Verification items for the finished model (mm, model axes). Face numbers are marked on the shaded views. A direction names the side the tool comes from. Round coordinates to 2 decimals unless told otherwise and drop trailing zeros. Write each loop counter-clockwise with the first axis right and the second up, starting at its lowest first coordinate (ties: lowest second). Pieces come first, ordered by that corner, then holes. Notation, with made-up numbers: (81.5, -37.5) -> (133.5, -37.5) arc R20 cw to (133.5, -0.5) -> close; hole circle Ø3 at (66, 57.5). An arc over 180 degrees is marked (long way). Answer as a JSON object with one key per item and string values. Group by question number.
(1) Sectioned sample at B-B on x = 29. Record the cut outline in (y, z).
(2) Scan lines: L1, parallel to X at y = -41, z = 7; L2, parallel to Y at x = -60, z = 83.5; L3, parallel to Y at x = 21, z = 69. Record each from-to range of solid material in increasing order. Write a range as from..to.
(3) Gauge pin test, flat ends, axial feed: pin 1 Ø3 at (y, z) = (-21, 25.5) entering from +X; pin 2 Ø2 at (y, z) = (14, 122.5) entering from -X; pin 3 Ø4 at (x, y) = (8, 21.5) entering from -Z; pin 4 Ø1 at (x, z) = (21.5, 25.5) entering from -Y. Record the tip position at first contact, or that the pin passes through.
(4) Sectioned sample at A-A on z = 19. Record the cut outline in (x, y).
(5) Set-up check for the marked faces 1, 2 and 3: record each of +Z, -Z, +X, -X, +Y, -Y from which the full face is reachable in a straight line by a thin tool's end or side.
(6) Sectioned sample at C-C on y = 39. Record the cut outline in (x, z).
```python
from build123d import *

# Parameters (mm, degrees)
F1_DEPTH = 146.05
F2_R     = 6.35


with BuildPart() as f1:
    # F0 (on Top) → F1 (new body)
    with BuildSketch(Plane.XY):
        Polygon((0, -52.3875), (0, -17.4625), (69.85, -17.4625), (69.85, 52.3875), (0, 52.3875), (0, 17.4625), (-69.85, 17.4625), (-69.85, -52.3875), align=None)
    extrude(amount=F1_DEPTH)

    # F2
    f2_edges = [f1.edges().sort_by_distance(p)[0] for p in [
        (-34.925, -52.3875, 146.05),
        (0, -34.925, 146.05),
        (34.925, -17.4625, 146.05),
        (69.85, 17.4625, 146.05),
        (34.925, 52.3875, 146.05),
        (0, 34.925, 146.05),
        (-34.925, 17.4625, 146.05),
        (-69.85, -17.4625, 146.05),
        (-69.85, -52.3875, 73.025),
        (0, -52.3875, 73.025),
        (-34.925, -52.3875, 0),
        (0, -17.4625, 73.025),
        (69.85, -17.4625, 73.025),
        (34.925, -17.4625, 0),
        (69.85, 52.3875, 73.025),
        (69.85, 17.4625, 0),
        (0, 52.3875, 73.025),
        (34.925, 52.3875, 0),
        (0, 17.4625, 73.025),
        (0, 34.925, 0),
        (-69.85, 17.4625, 73.025),
        (-34.925, 17.4625, 0),
        (-69.85, -17.4625, 0),
        (0, -34.925, 0),
    ]]
    fillet(f2_edges, radius=F2_R)


solid = f1.part
```
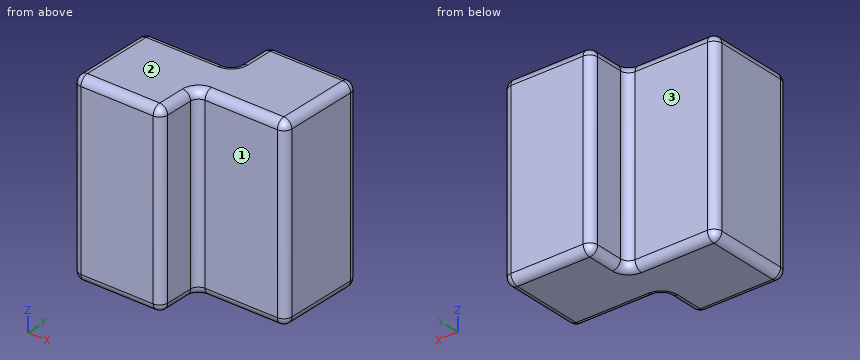
Computed values:
{
 "1": {"outline": "(-17.46, 6.35) arc R6.35 ccw to (-11.11, 0) -> (46.04, 0) arc R6.35 ccw to (52.39, 6.35) -> (52.39, 139.7) arc R6.35 ccw to (46.04, 146.05) -> (-11.11, 146.05) arc R6.35 ccw to (-17.46, 139.7) -> close"},
 "2": {"L1": "-69.85..0", "L2": "-52.39..17.46", "L3": "-17.46..52.39"},
 "3": {"pin 1": "x = 1.69", "pin 2": "x = -69.56", "pin 3": "z = 0", "pin 4": "y = -17.46"},
 "4": {"outline": "(-69.85, -46.04) arc R6.35 ccw to (-63.5, -52.39) -> (-6.35, -52.39) arc R6.35 ccw to (0, -46.04) -> (0, -23.81) arc R6.35 cw to (6.35, -17.46) -> (63.5, -17.46) arc R6.35 ccw to (69.85, -11.11) -> (69.85, 46.04) arc R6.35 ccw to (63.5, 52.39) -> (6.35, 52.39) arc R6.35 ccw to (0, 46.04) -> (0, 23.81) arc R6.35 cw to (-6.35, 17.46) -> (-63.5, 17.46) arc R6.35 ccw to (-69.85, 11.11) -> close"},
 "5": {"face 1": "+Z, -Z, +X, -Y", "face 2": "+Z, +X, -X, +Y, -Y", "face 3": "+Z, -Z, -X, +Y"},
 "6": {"outline": "(0, 6.35) arc R6.35 ccw to (6.35, 0) -> (63.5, 0) arc R6.35 ccw to (69.85, 6.35) -> (69.85, 139.7) arc R6.35 ccw to (63.5, 146.05) -> (6.35, 146.05) arc R6.35 ccw to (0, 139.7) -> close"}
}
